For this review, use the dimensioned drawing (mm, ordinates from the lowest corner) and the shaded views. A direction names the side the tool comes from. Give positions to 0.01 mm unless a question says otherwise; leave off trailing zeros. Order: outer loops, then holes, each group sorted by start corner. A loop starts at its lowest first (then second) coordinate and runs counter-clockwise, first axis right, second up.
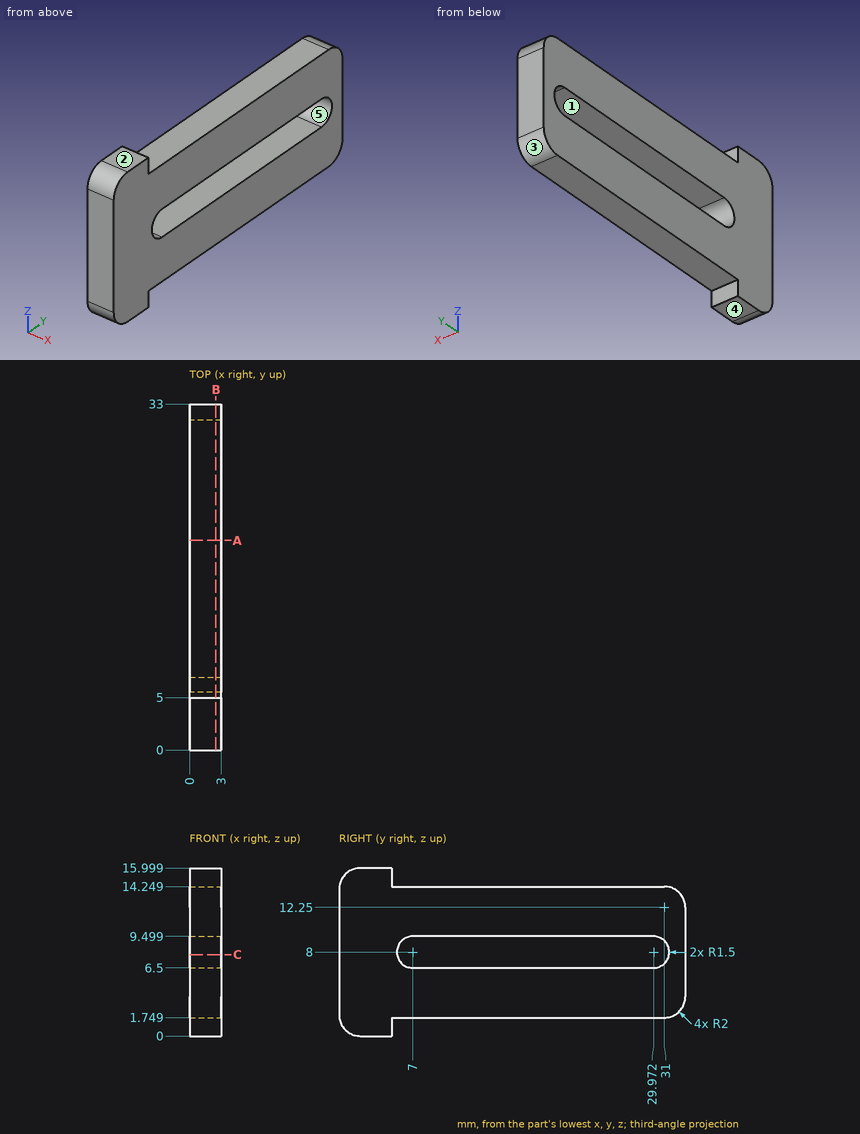
1. For pin 1 (1.5 mm diameter, centred on x = 1, y = 16, fed in from -Z); pin 2 (1.5 mm diameter, centred on x = 1, y = 19.5, fed in from +Z); pin 3 (0.5 mm diameter, centred on x = 2, z = 15.5, fed in from +Y), all flat-tipped, find the tip position at first contact; note any pin that passes through.
Recorded:
pin 1: stops at z = 1.75
pin 2: stops at z = 14.25
pin 3: stops at y = 5
2. For line 1 along Z through (x, y) = (1.45, 21); line 2 along Y through (x, z) = (1.55, 8), list the stretches that pass through material, from the lowest coordinate up.
Recorded:
line 1: z = 1.75 to 6.5, 9.5 to 14.25
line 2: y = 0 to 5.5, 31.47 to 33
3. Machinability: for the marked faces 1 and 2, which of the approach directions +Z, -Z, +X, -X, +Y, -Y give a long, thin tool a straight path to every point of the face, cutting with its end or side? Answer none if there is none.
Recorded:
face 1: +X, -X
face 2: +Z, +X, -X, +Y, -Y
4. Draft analysis for pull direction Y (two halves, no side actions). For the marked faces 3, 4 and 5, state which applies: pulls with the +Y half, pulls with the -Y half, needs draft (parallel to the pull), parting line crosses it, or undercut.
Recorded:
face 3: pulls with the +Y half
face 4: needs draft
face 5: undercut
5. Take a section at B-B (x = 2.5). State the section outline as (y, z) points.
Recorded:
outline: (0, 2) arc R2 ccw to (2, 0) - (5, 0) - (5, 1.75) - (31, 1.75) arc R2 ccw to (33, 3.75) - (33, 12.25) arc R2 ccw to (31, 14.25) - (5, 14.25) - (5, 16) - (2, 16) arc R2 ccw to (0, 14) - close; hole (6.97, 6.5) - (29.97, 6.5) arc R1.5 ccw to (29.97, 9.5) - (6.97, 9.5) arc R1.5 ccw to start
6. Take a section at A-A (y = 20). State the section outline as (x, z) points.
Recorded:
outline: (0, 1.75) - (3, 1.75) - (3, 6.5) - (0, 6.5) - close; (0, 9.5) - (3, 9.5) - (3, 14.25) - (0, 14.25) - close
7. Take a section at C-C (z = 7.75). State the section outline as (x, y) points.
Recorded:
outline: (0, 0) - (3, 0) - (3, 5.52) - (0, 5.52) - close; (0, 31.45) - (3, 31.45) - (3, 33) - (0, 33) - close
